```python
from build123d import *

# Parameters (mm, degrees)
SKETCH3_R           = 4
SKETCH3_R_2         = 3.175
BOSS_EXTRUDE1_DEPTH = 6.35


with BuildPart() as part:
    # Sketch3 → Boss-Extrude1 (new body)
    with BuildSketch(Plane.XY):
        with BuildLine():
            ThreePointArc((-54.344755215, 14.159551399), (-91.363790432, 41.595955293), (-133.974414464, 24.060278895))
            Line((-133.974414464, 24.060278895), (-211.005412605, -73.916742383))
            ThreePointArc((-211.005412605, -73.916742383), (-211.144018552, -88.650897892), (-196.929213693, -92.530829979))
            Line((-196.929213693, -92.530829979), (-103.422476429, -54.04933414))
            ThreePointArc((-103.422476429, -54.04933414), (-97.145595861, -52.808695879), (-90.869059624, -54.05107498))
            Line((-90.869059624, -54.05107498), (2.122974069, -92.350913963))
            ThreePointArc((2.122974069, -92.350913963), (16.383743715, -88.415214787), (16.111301916, -73.623830322))
            Line((16.111301916, -73.623830322), (-53.413545275, 12.636035393))
            ThreePointArc((-53.413545275, 12.636035393), (-53.928639798, 13.36754418), (-54.344755215, 14.159551399))
        make_face()
        with BuildLine():
            ThreePointArc((-94.365331084, -37.471342529), (-94.782391681, -37.306590994), (-95.20914515, -37.168880842))
            Line((-95.20914515, -37.168880842), (-105.570837866, -34.188121867))
            ThreePointArc((-105.570837866, -34.188121867), (-122.920802355, 11.370636159), (-74.330134016, 15.316349154))
            Line((-74.330134016, 15.316349154), (-54.078953085, -7.541638988))
            ThreePointArc((-54.078953085, -7.541638988), (-54.00749546, -7.623730088), (-53.937484416, -7.707058323))
            Line((-53.937484416, -7.707058323), (-12.08621589, -58.41284178))
            ThreePointArc((-12.08621589, -58.41284178), (-11.885929876, -67.212968778), (-20.394707026, -69.467533275))
            Line((-20.394707026, -69.467533275), (-94.365331084, -37.471342529))
        make_face(mode=Mode.SUBTRACT)
        with BuildLine():
            ThreePointArc((-172.528906448, -72.18914022), (-180.908159839, -69.902022358), (-180.826455281, -61.216625426))
            Line((-180.826455281, -61.216625426), (-155.117076369, -28.516434264))
            ThreePointArc((-155.117076369, -28.516434264), (-149.40547172, -25.801135391), (-143.78928279, -28.708659687))
            Line((-143.78928279, -28.708659687), (-131.33676671, -45.703813477))
            ThreePointArc((-131.33676671, -45.703813477), (-130.226967626, -51.831800551), (-134.367011458, -56.484102848))
            Line((-134.367011458, -56.484102848), (-172.528906448, -72.18914022))
        make_face(mode=Mode.SUBTRACT)
        with Locations((-130.919350653, -24.396060329)):
            Circle(SKETCH3_R, mode=Mode.SUBTRACT)
        with Locations((-97.144359905, -43.896060329)):
            Circle(SKETCH3_R, mode=Mode.SUBTRACT)
        with Locations((-130.919350653, 14.603939671)):
            Circle(SKETCH3_R, mode=Mode.SUBTRACT)
        with Locations((-63.369369158, 14.603939671)):
            Circle(SKETCH3_R, mode=Mode.SUBTRACT)
        with Locations((-97.144359905, 34.103939671)):
            Circle(SKETCH3_R, mode=Mode.SUBTRACT)
        with Locations((6.717643784, -81.195052938)):
            Circle(SKETCH3_R_2, mode=Mode.SUBTRACT)
        with Locations((-201.520789163, -81.373695056)):
            Circle(SKETCH3_R_2, mode=Mode.SUBTRACT)
    extrude(amount=BOSS_EXTRUDE1_DEPTH)


solid = part.part
```
CAD build for the part. Positions are in the model's coordinates, mm. A direction names the side the tool comes from. Coordinates: 2 decimals unless noted, no trailing zeros. Loops run counter-clockwise (first coordinate to the right, second up) from the corner with the lowest first, then second, coordinate; pieces in that order, holes last. Notation, with made-up numbers: (72.5, 11.5) - (115.5, 11.5) arc R6 ccw to (115.5, 15.5) - close; hole circle Ø4 at (12.25, 16). An arc over 180 degrees is marked (long way). Return JSON: item names as keys, results as strings.
1. Band-saw the part on A-A (x = -26.5). Give the cut face in (y, z), and give its area (3 significant figures).
Result:
{"outline": "(-80.56, 0) - (-66.83, 0) - (-66.83, 6.35) - (-80.56, 6.35) - close; (-40.95, 0) - (-20.76, 0) - (-20.76, 6.35) - (-40.95, 6.35) - close", "area": "215 mm2"}
2. Probe L1, parallel to Y at x = -61, z = 6.25; L2, parallel to X at y = -80.5, z = 0.5; L3, parallel to X at y = 13.5, z = 4.5. List the from-to ranges inside material, lowest first. Write a range as from..to.
Result:
{"L1": "y = -66.35..-51.9, 0.27..11.38, 17.83..24.91", "L2": "x = -213.55..-204.57, -198.47..-167.7, -26.65..3.62, 9.82..18.76", "L3": "x = -142.28..-134.76, -127.07..-121.45, -72.72..-67.21, -59.52..-54.01"}
3. Band-saw the part on B-B (y = 0.5). Give the cut face in (x, z).
Result:
{"outline": "(-152.5, 0) - (-127.14, 0) - (-127.14, 6.35) - (-152.5, 6.35) - close; (-61.2, 0) - (-43.63, 0) - (-43.63, 6.35) - (-61.2, 6.35) - close"}
4. Band-saw the part on C-C (z = 2.5). State how many separate pieces and enclosed holes the cut face has, and give its area (3 significant figures).
Result:
{"separate pieces": "1", "enclosed holes": "9", "area": "8,800 mm2"}
5. 3-axis set-ups, long thin cutter, end or side, ignore diameter. For faces 1 (the flat face through (-45.024, -72.933, 3.131)), 2 (the cylindrical face through (-149.5, -25.8, 3.1)): which of +Z, -Z, +X, -X, +Y, -Y reach the whole face in a straight line?
Result:
{"face 1": "+Z, -Z, -Y", "face 2": "+Z, -Z"}
6. Drop flat-ended pins along their axis: pin 1 (10.5 mm diameter, centred on x = -130.92, y = 14.6, fed in from +Z); pin 2 (1.5 mm diameter, centred on x = -53.5, z = 1.5, fed in from -Y); pin 3 (1 mm diameter, centred on x = -71.5, z = 4.5, fed in from +Y); pin 4 (1 mm diameter, centred on y = 1.5, z = 5.5, fed in from +X) (3 decimals). Give the stop position or say it passes through.
Result:
{"pin 1": "stops at z = 6.35", "pin 2": "stops at y = -69.75", "pin 3": "stops at y = 34.63", "pin 4": "stops at x = -44.035"}
7. Mould opens along X. For faces 3 (the flat face through (-18.164, -31.098, 3.131)), 4 (the cylindrical face through (-11.81, -67.11, 3.13)), 5 (the cylindrical face through (-90.7, 41.51, 3.13)), 6 (the flat face through (-171.95, -24.24, 3.13)) say: released by +X, released by -X, zero draft, split by the parting line, or undercut.
Result:
{"face 3": "released by +X", "face 4": "undercut", "face 5": "split by the parting line", "face 6": "released by -X"}
